from build123d import *

# Parameters (mm, degrees)
SKETCH1_R                 = 10
BOSS_EXTRUDE1_DEPTH       = 60
SKETCH3_W                 = 30
SKETCH3_H                 = 30
BOSS_EXTRUDE2_DEPTH       = 5
F_4_0MM_DOWEL_HOLE1_D     = 4
F_4_0MM_DOWEL_HOLE1_DEPTH = 35
F_4_0MM_DOWEL_HOLE1_TIP   = 1.201721238


with BuildPart() as part:
    # Sketch1 → Boss-Extrude1 (new body)
    with BuildSketch(Plane.XY):
        with Locations(Location((0, 0, 0), (0, 0, 180))):
            Circle(SKETCH1_R)
    extrude(amount=BOSS_EXTRUDE1_DEPTH)

    # Sketch3 → Boss-Extrude2 (add)
    with BuildSketch(Plane(origin=(0, 0, 0), x_dir=(-1, 0, 0), z_dir=(0, 0, -1))):
        Rectangle(SKETCH3_W, SKETCH3_H)
    extrude(amount=-BOSS_EXTRUDE2_DEPTH)

    # Ø4.0mm Dowel Hole1
    with Locations(Plane(origin=(-10.433527311, 10.715968246, 5), x_dir=(1, 0, 0), z_dir=(0, 0, 1))):
        with Locations((0, 0), (21.120601919, -20.899829076)):
            Hole(F_4_0MM_DOWEL_HOLE1_D / 2, depth=F_4_0MM_DOWEL_HOLE1_DEPTH)
            with Locations((0, 0, -(F_4_0MM_DOWEL_HOLE1_DEPTH + F_4_0MM_DOWEL_HOLE1_TIP / 2))):  # 118° drill point
                Cone(0, F_4_0MM_DOWEL_HOLE1_D / 2, F_4_0MM_DOWEL_HOLE1_TIP, mode=Mode.SUBTRACT)


solid = part.part
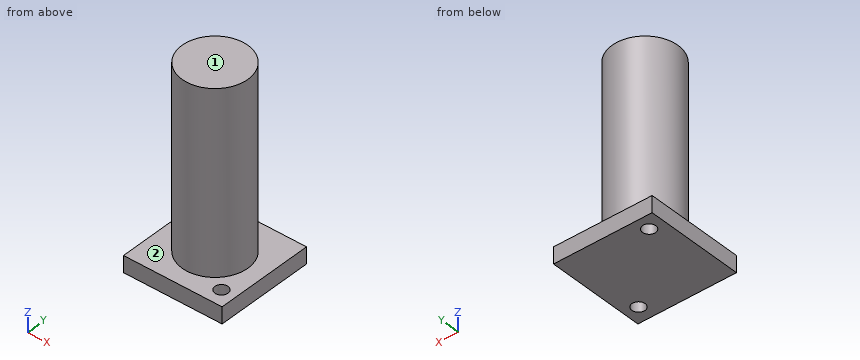
Design review of the part built by this model. Coordinates are the model's own, in mm. Face numbers are marked on the shaded views. A direction names the side the tool comes from. Coordinates: 2 decimals unless noted, no trailing zeros. Order: outer loops, then holes, each group sorted by start corner. A loop starts at its lowest first (then second) coordinate and runs counter-clockwise, first axis right, second up. Notation, with made-up numbers: (29, -23) -> (64, -23) arc R21 cw to (64, 8) -> close; hole circle Ø10 at (1.5, 54.5). An arc over 180 degrees is marked (long way). One line per item, written item: value.
1) Clearance check with flat-ended pins moving along their axes: P1, Ø8, axis at x = 10.5, y = -9, coming from the +Z side; P2, Ø1.5, axis at y = -4, z = 26, coming from the +X side; P3, Ø6, axis at x = 3.5, z = 20.5, coming from the +Y side; P4, Ø4.5, axis at x = 10.69, y = -10.18, coming from the +Z side. State where each tip first meets the part, or that it passes through.
Output values:
P1: stops at z = 60
P2: stops at x = 9.46
P3: stops at y = 9.99
P4: stops at z = 5
2) To check wall thickness, follow probe 1 along Z at (x, y) = (-5, -10); probe 2 along X at (y, z) = (0.5, 55); probe 3 along Y at (x, z) = (7.25, 20). State the ranges of each line that lie inside material, in increasing order. Write a range as [from, to].
Output values:
probe 1: z = [0, 5]
probe 2: x = [-9.99, 9.99]
probe 3: y = [-6.89, 6.89]
3) We need section C-C, the plane z = 36. Give the boundary of the cut face in (x, y).
Output values:
outline: circle Ø20 at (0, 0)
4) Machinability: for the marked faces 1 and 2, which of the approach directions +Z, -Z, +X, -X, +Y, -Y give a long, thin tool a straight path to every point of the face, cutting with its end or side? Answer none if there is none.
Output values:
face 1: +Z, +X, -X, +Y, -Y
face 2: +Z
5) We need section A-A, the plane y = 0. Give the boundary of the cut face in (x, z), then the cut area to 3 significant figures.
Output values:
outline: (-15, 0) -> (15, 0) -> (15, 5) -> (10, 5) -> (10, 60) -> (-10, 60) -> (-10, 5) -> (-15, 5) -> close
area: 1,250 mm2
